The model under review builds one solid part; all positions refer to its coordinate system, in mm. A direction names the side the tool comes from. Give positions to 0.01 mm unless a question says otherwise; leave off trailing zeros. Loops run counter-clockwise (first coordinate to the right, second up) from the corner with the lowest first, then second, coordinate; pieces in that order, holes last. Notation, with made-up numbers: (0.25, 16.25) - (14.25, 16.25) arc R21 cw to (14.25, 21.25) - close; hole circle Ø11 at (-26, 6.25). An arc over 180 degrees is marked (long way). Answer as a JSON object with one key per item and string values.
from build123d import *

# Parameters (mm, degrees)
PAD049_DEPTH = 6
PAD050_DEPTH = 6
PAD051_DEPTH = 18
PAD043_DEPTH = 20
PAD041_DEPTH = 33
PAD042_DEPTH = 20
PAD040_DEPTH = 33


with BuildPart() as pad049:
    # Sketch053 → Pad049 (new body)
    with BuildSketch(Plane.XZ.offset(4)):
        Polygon((-22.876627, -50.458862), (-2.795745, -40.418423), (3.522805, -28.90654), (-39.408733, -32.801537), align=None)
    extrude(amount=PAD049_DEPTH)


with BuildPart() as pad050:
    # Sketch054 → Pad050 (new body)
    with BuildSketch(Plane.XZ.offset(24)):
        Polygon((-22.876627, -50.458862), (-2.795745, -40.418423), (3.522805, -28.90654), (-39.408733, -32.801537), align=None)
    extrude(amount=PAD050_DEPTH)


with BuildPart() as pad051:
    # Sketch055 → Pad051 (new body)
    with BuildSketch(Plane.XZ.offset(3.5)):
        Polygon((26.854265, -42.508881), (4.226509, -42.508881), (-12.077076, -26.263317), (32.65625, -19.126871), align=None)
    extrude(amount=PAD051_DEPTH)


with BuildPart() as pad043:
    # Sketch047 → Pad043 (new body)
    with BuildSketch(Plane(origin=(10, -7, 0), x_dir=(1, 0, 0), z_dir=(0, -1, 0))):
        Polygon((12.921668, -76.043343), (12.921668, -72.681298), (10.907037, -71.064545), (12.949577, -67.987406), (17.894252, -67.987406), (19.953335, -71.012405), (17.993304, -72.648705), (17.981073, -76.043343), align=None)
    extrude(amount=PAD043_DEPTH)


with BuildPart() as pad041:
    # Sketch045 → Pad041 (new body)
    with BuildSketch(Plane.XZ):
        Polygon((31.922119, -73.764191), (34.715668, -84.347412), (31.00419, -84.347412), (29.994871, -83.010223), (29.004835, -82.997353), (29.97435, -84.356453), (27.001257, -84.356453), (25.99424, -83.013763), (24.977634, -83.013763), (26.003832, -84.375633), (23.007538, -84.375633), (22.019703, -83.023636), (20.974325, -83.023636), (22.000523, -84.366325), (19.017838, -84.366325), (17.99164, -83.004456), (16.984625, -83.004456), (18.00123, -84.366325), (15.032244, -84.366325), (14.013124, -83.020378), (12.982291, -83.020378), (14.00141, -84.379204), (12.681671, -84.379204), (4.650895, -73.764191), align=None)
    extrude(amount=PAD041_DEPTH)


with BuildPart() as fusion011:
    # Sketch046 → Pad042 (new body)
    with BuildSketch(Plane(origin=(-4, -7, 0), x_dir=(1, 0, 0), z_dir=(0, -1, 0))):
        Polygon((12.921668, -76.043343), (12.921668, -72.681298), (10.907037, -71.064545), (12.949577, -67.987406), (17.894252, -67.987406), (19.953335, -71.012405), (17.993304, -72.648705), (17.981073, -76.043343), align=None)
    extrude(amount=PAD042_DEPTH)

    # Fusion010: union Pad041
    add(pad041.part)

    # Fusion011: union Pad043
    add(pad043.part)


with BuildPart() as cut018:
    # Sketch043 → Pad040 (new body)
    with BuildSketch(Plane(origin=(-15, 0, -10), x_dir=(0.819152, 0, 0.573576), z_dir=(0, -1, 0))):
        Polygon((-26.184557, -19.824878), (-21.536683, -15.979609), (13.963177, -33.561758), (16.497322, -39.355457), (1.912507, -79.157962), (-20.506964, -63.527428), align=None)
    extrude(amount=PAD040_DEPTH)

    # Cut010: cut Fusion011
    add(fusion011.part, mode=Mode.SUBTRACT)

    # Cut016: cut Pad051
    add(pad051.part, mode=Mode.SUBTRACT)

    # Cut017: cut Pad050
    add(pad050.part, mode=Mode.SUBTRACT)

    # Cut018: cut Pad049
    add(pad049.part, mode=Mode.SUBTRACT)


with BuildPart() as part_mirroring019:
    # Part__Mirroring019: instance of Cut018
    add(cut018.part.mirror(Plane(origin=(0, 0, 0), x_dir=(0, -1, 0), z_dir=(1, 0, 0))))


with BuildPart() as part_mirroring019_1:
    # Part__Mirroring019 placement: moved
    add(part_mirroring019.part.moved(Location((76, 0, 0))))


solid = part_mirroring019_1.part
Q1. Clearance check with flat-ended pins moving along their axes: pin 1 Ø4 at (x, y) = (91, -29) entering from -Z; pin 2 Ø1 at (x, y) = (50.5, -24) entering from -Z; pin 3 Ø9 at (x, y) = (59.5, -11.5) entering from -Z. State where each tip first meets the part, or that it passes through.
Results:
{"pin 1": "stops at z = -54.48", "pin 2": "stops at z = -67.99", "pin 3": "stops at z = -73.76"}
Q2. Consider section D-D, the plane x = 78. State the section outline as (y, z) points, plus the area to 3 significant figures.
Results:
{"outline": "(-33, -66.53) - (0, -66.53) - (0, -32.17) - (-3.5, -32.17) - (-3.5, -36.3) - (-4, -36.3) - (-4, -38.97) - (-10, -38.97) - (-10, -36.3) - (-21.5, -36.3) - (-21.5, -32.17) - (-24, -32.17) - (-24, -38.97) - (-30, -38.97) - (-30, -32.17) - (-33, -32.17) - close", "area": "1,000 mm^2"}
Q3. To check wall thickness, follow probe 1 along Y at (x, z) = (69, -40); probe 2 along X at (y, z) = (-13, -71); probe 3 along Z at (x, y) = (62.5, -12). State the ranges of each line that lie inside material, in increasing order. Write a range as [from, to].
Results:
{"probe 1": "y = [-33, -21.5], [-3.5, 0]", "probe 2": "x = [44.76, 46.06], [55.05, 60.06], [69.05, 73.92]", "probe 3": "z = [-67.99, -42.51]"}
Q4. Consider section B-B, the plane x = 96. State the section outline as (y, z) points, plus the area to 3 significant figures.
Results:
{"outline": "(-33, -46.82) - (-30, -46.82) - (-30, -34.91) - (-33, -34.91) - close; (-24, -46.82) - (-10, -46.82) - (-10, -34.91) - (-24, -34.91) - close; (-4, -46.82) - (0, -46.82) - (0, -34.91) - (-4, -34.91) - close", "area": "250 mm^2"}
Q5. The part is to be moulded in two halves that separate along Z. For faces 1 (the face through (54.09, -16.86, -69.55)), 2 (the face through (88, -24, -40)), 3 (the face through (77.937, -6.958, -38.855)), say which applies: +Z half, -Z half, draft (parallel to the pull), parting line (faces both ways), or undercut.
Results:
{"face 1": "undercut", "face 2": "draft", "face 3": "+Z half"}
Q6. For faces 4 (the face through (51, -17, -67.987)), 5 (the face through (61.09, -16.86, -69.48)), 6 (the face through (88, -30, -40)), list the 3-axis set-ups (+Z, -Z, +X, -X, +Y, -Y) from which the entire face can be reached by the end or side of a thin tool; tool diameter is ignored.
Results:
{"face 4": "-Z", "face 5": "none", "face 6": "+Z, +X"}
Q7. Consider section C-C, the plane z = -39.5. State the section outline as (x, y) points.
Results:
{"outline": "(53.13, -33) - (100.59, -33) - (100.59, -30) - (78.29, -30) - (78.29, -24) - (100.59, -24) - (100.59, -10) - (78.29, -10) - (78.29, -4) - (100.59, -4) - (100.59, 0) - (53.13, 0) - (53.13, -3.5) - (74.79, -3.5) - (74.79, -21.5) - (53.13, -21.5) - close"}
